The listing builds one solid part. Answer for the finished solid, in the listing's coordinates (mm). Face numbers are marked on the shaded views. A direction names the side the tool comes from. Round coordinates to 2 decimals unless told otherwise and drop trailing zeros. Write each loop counter-clockwise with the first axis right and the second up, starting at its lowest first coordinate (ties: lowest second). Pieces come first, ordered by that corner, then holes. Notation, with made-up numbers: (16.25, 17) - (26.25, 17) arc R14 cw to (26.25, 35) - close; hole circle Ø10 at (3.5, 22.5). An arc over 180 degrees is marked (long way). Return JSON: item names as keys, results as strings. Group by question number.
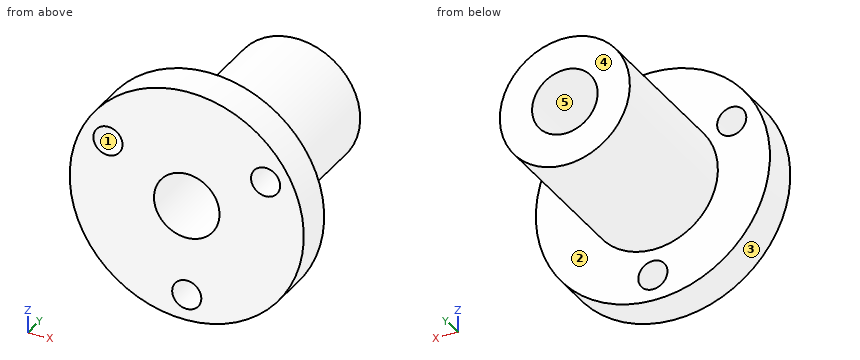
Autodesk Inventor part; units mm, degrees
ref_plane "YZ Plane" through (0, 0, 0) normal (1, 0, 0) x (0, 1, 0)
ref_plane "XZ Plane" through (0, 0, 0) normal (0, 1, 0) x (-1, 0, 0)
ref_plane "XY Plane" through (0, 0, 0) normal (0, 0, 1) x (1, 0, 0)
sketch "Sketch1" plane through (0, 0, 0) normal (1, 0, 0) x (0, 1, 0)
  line L0 (0, 0) -> (25.4, 0)
  line L1 (25.4, 0) -> (25.4, -7.9375)
  line L2 (25.4, -7.9375) -> (4.7752, -7.9375)
  line L3 (4.7752, -7.9375) -> (4.7752, -14.2875)
  line L4 (4.7752, -14.2875) -> (0, -14.2875)
  line L5 (0, -14.2875) -> (0, 0)
  dimension "d0" = 25.4
  dimension "d1" = 4.7752
  dimension "d2" = 7.9375
  dimension "d3" = 14.2875
revolve "Revolution1" add sketch "Sketch1" angle 360 about axis through (0, 0, 0) along (0, 1, 0)
hole "Hole1" at (0, 25.4, 0) direction (0, -1, 0) diameter 8.001 end through all
sketch "Sketch2" plane through (0, 4.7752, 0) normal (0, 1, 0) x (1, 0, 0)
  circle A0 centre (0, 0) radius 11.1125
  line L0 (-9.6237, -5.5562) -> (0, 0)
  line L1 (0, 0) -> (9.6237, -5.5562)
  line L2 (0, 0) -> (0, 11.1125)
  point P0 (-9.6237, -5.5562)
  dimension "d16" = 120
  dimension "d17" = 120
  dimension "d18" = 22.225
hole "Hole2" at (0, 4.7752, -11.1125) at (-9.6237, 4.7752, 5.5562) at (9.6237, 4.7752, 5.5562) direction (0, -1, 0) diameter 3.556 end through all
properties part number "Lead_Screw_Flange_Nut"
(1) Find section C-C (x = -3.5). Write down the section's boundary in (y, z), plus the area to 3 significant figures.
(2) Determine the mould class of the marked faces 3, 4 and 5 for opening direction Z: +Z half, -Z half, draft (parallel to the pull), parting line (faces both ways), or undercut.
(3) For the marked faces 1 and 2, determine the directions among +Z, -Z, +X, -X, +Y, -Y from which every point of the face is accessible in a straight line to the end or side of a thin tool.
(4) Consider line 1 (Z direction, x = 0, y = 2.4); line 2 (Z direction, x = -0.25, y = 17.75); line 3 (Y direction, x = 12.5, z = -4.5). Determine where each line is inside the solid, lowest interval first.
(5) Flat-ended cylindrical pins translate along their axes: pin 1 (3 mm diameter, centred on x = 9.62, z = 5.56, fed in from -Y); pin 2 (5 mm diameter, centred on x = -7.5, z = -11.5, fed in from +Y); pin 3 (5 mm diameter, centred on x = 9.5, y = 5.5, fed in from -Z); pin 4 (3 mm diameter, centred on x = 5, y = 22.5, fed in from -Z). Find the tip coordinate at first contact, or state that the pin passes through.
(6) Find section A-A (x = 0). Write down the section's boundary in (y, z), plus the area to 3 significant figures.
(7) Find section D-D (y = 11.5). Write down the section's boundary in (x, z) (1 decimal), plus the area to 3 significant figures.
(8) Find section B-B (z = 0). Write down the section's boundary in (x, y), plus the area to 3 significant figures.
Check sheet entries:
{
 "1": {"outline": "(0, -13.85) - (4.78, -13.85) - (4.78, -7.12) - (25.4, -7.12) - (25.4, -1.94) - (0, -1.94) - close; (0, 1.94) - (25.4, 1.94) - (25.4, 7.12) - (4.78, 7.12) - (4.78, 13.85) - (0, 13.85) - close", "area": "328 mm^2"},
 "2": {"face 3": "parting line", "face 4": "draft", "face 5": "undercut"},
 "3": {"face 1": "+Y, -Y", "face 2": "+Y"},
 "4": {"line 1": "z = -14.29 to -12.89, -9.33 to -4, 4 to 14.29", "line 2": "z = -7.93 to -3.99, 3.99 to 7.93", "line 3": "y = 0 to 4.78"},
 "5": {"pin 1": "passes through", "pin 2": "stops at y = 4.78", "pin 3": "stops at z = -12.39", "pin 4": "stops at z = -7.12"},
 "6": {"outline": "(0, -14.29) - (4.78, -14.29) - (4.78, -12.89) - (0, -12.89) - close; (0, -9.33) - (4.78, -9.33) - (4.78, -7.94) - (25.4, -7.94) - (25.4, -4) - (0, -4) - close; (0, 4) - (25.4, 4) - (25.4, 7.94) - (4.78, 7.94) - (4.78, 14.29) - (0, 14.29) - close", "area": "244 mm^2"},
 "7": {"outline": "circle Ø15.9 at (0, 0); hole circle Ø8 at (0, 0)", "area": "148 mm^2"},
 "8": {"outline": "(-14.29, 0) - (-4, 0) - (-4, 25.4) - (-7.94, 25.4) - (-7.94, 4.78) - (-14.29, 4.78) - close; (4, 0) - (14.29, 0) - (14.29, 4.78) - (7.94, 4.78) - (7.94, 25.4) - (4, 25.4) - close", "area": "261 mm^2"}
}
